from build123d import *

# Parameters (mm, degrees)
F0_R     = 1
F1_DEPTH = 22.5
F2_W     = 4
F2_H     = 5.5
F3_DEPTH = 12.5
F4_W     = 4
F4_H     = 2.8967225653
F4_H_2   = 2.6032774347
F5_DEPTH = 12.5


with BuildPart() as f1:
    # F0 (on Right) → F1 (new body)
    with BuildSketch(Plane.YZ):
        with BuildLine():
            Line((-2.25, 6.0981554588), (-2.4978658434, 0.1032774347))
            ThreePointArc((-2.4978658434, 0.1032774347), (0, -2.5), (2.4978658434, 0.1032774347))
            Line((2.4978658434, 0.1032774347), (2.25, 6.0981554588))
            Line((2.25, 6.0981554588), (-2.25, 6.0981554588))
        make_face()
        Circle(F0_R, mode=Mode.SUBTRACT)
    extrude(amount=F1_DEPTH)

    # F2 (on Front) → F3 (intersect, symmetric)
    with BuildSketch(Plane.XZ):
        Polygon((18.25, 6.0981554588), (4.25, 6.0981554588), (4.25, 4.5981554588), (0.5, 4.5981554588), (0, -2.5), (5.25, -2.5), (5.25, 3), (9.25, 3), (9.25, -2.5), (13.25, -2.5), (13.25, 3), (17.25, 3), (17.25, -2.5), (22.0024140141, -2.5), (22.0008491054, 4.5981554588), (18.25, 4.5981554588), align=None)
        Polygon((5.25, -2.5), (0, -2.5), (5.25, -3.4987433143), align=None)
        Polygon((21.3468169383, -4.6197534539), (22.0024140141, -2.5), (17.25, -2.5), (17.25, -4.6197534539), align=None)
        with Locations((7.25, 0.25)):
            Rectangle(F2_W, F2_H)
        with Locations((15.25, 0.25)):
            Rectangle(F2_W, F2_H)
        Polygon((13.25, -2.5), (9.25, -2.5), (9.25, -3.4987433143), (13.25, -4.6197534539), align=None)
    extrude(amount=F3_DEPTH, both=True, mode=Mode.INTERSECT)

    # F4 (on Front) → F5 (cut, symmetric)
    with BuildSketch(Plane.XZ):
        with Locations((7.25, 1.5516387174)):
            Rectangle(F4_W, F4_H)
        Polygon((9.25, -2.5), (5.25, -2.5), (5.25, -7), (17.25, -7), (17.25, -2.5), (13.25, -2.5), (13.25, -5), (9.25, -5), align=None)
        with Locations((7.25, -1.1983612826)):
            Rectangle(F4_W, F4_H_2)
        with Locations((15.25, 1.5516387174)):
            Rectangle(F4_W, F4_H)
        with Locations((15.25, -1.1983612826)):
            Rectangle(F4_W, F4_H_2)
    extrude(amount=F5_DEPTH, both=True, mode=Mode.SUBTRACT)


solid = f1.part
CAD build for the part. Positions are in the model's coordinates, mm. A direction names the side the tool comes from. Round coordinates to 2 decimals unless told otherwise and drop trailing zeros. Loops run counter-clockwise (first coordinate to the right, second up) from the corner with the lowest first, then second, coordinate; pieces in that order, holes last.
(1) Which spindle directions (+Z, -Z, +X, -X, +Y, -Y) get a long thin tool onto all of the face, cutting with end or side? Do faces 1 (the flat face through (20, 0, 4.598)), 2 (the flat face through (10.94, 2.376, 3.059)), 3 (the flat face through (2, 0, 4.598)), 4 (the flat face through (15, 0, 3)), 5 (the cylindrical face through (11, 0, -1)). Say none if no direction does.
(2) Cut at B-B (z = 2). Give the cut face in (x, y), plus the area to 3 significant figures.
(3) Two-plate mould, pull along X, no slides. Class faces 6 (the flat face through (13.25, -1, 1)), 7 (the flat face through (18.25, 0, 5)), 8 (the cylindrical face through (20, 0, -1)), 9 (the flat face through (17.25, -1, 1)): +X half, -X half, draft (parallel to the pull), parting line (faces both ways), or undercut.
(4) Wall check: line 1 along X through (y, z) = (-0.45, -1); line 2 along Y through (x, z) = (2.5, 0); line 3 along Z through (x, y) = (2.6, 0). Give the ranges that are in metal, low to high.
(5) Drop flat-ended pins along their axis: pin 1 (3 mm diameter, centred on x = 7.5, y = 1, fed in from -Z); pin 2 (2.5 mm diameter, centred on y = 0, z = 0, fed in from -X); pin 3 (1.8 mm diameter, centred on y = 0, z = 0, fed in from -X); pin 4 (0.8 mm diameter, centred on y = -1, z = 5.5, fed in from +X). Give the stop position or say it passes through.
(6) Cut at D-D (y = 1.5). Give the cut face in (x, z), plus the area to 3 significant figures.
(7) Cut at A-A (y = 0.3). Give the cut face in (x, z), plus the area to 3 significant figures.
Findings below:
1. face 1: +Z, +X, +Y, -Y
1. face 2: +Z, +X, -X, +Y
1. face 3: +Z, -X, +Y, -Y
1. face 4: -Z, +Y, -Y
1. face 5: +X, -X
2. outline: (0.32, -2.42) - (5.25, -2.42) - (5.25, 2.42) - (0.32, 2.42) - close; (9.25, -2.42) - (13.25, -2.42) - (13.25, 2.42) - (9.25, 2.42) - close; (17.25, -2.42) - (22, -2.42) - (22, 2.42) - (17.25, 2.42) - close
2. area: 66.2 mm2
3. face 6: undercut
3. face 7: +X half
3. face 8: draft
3. face 9: undercut
4. line 1: x = 0.11 to 5.25, 9.25 to 13.25, 17.25 to 22
4. line 2: y = -2.5 to -1, 1 to 2.5
4. line 3: z = -2.5 to -1, 1 to 4.6
5. pin 1: stops at z = 3
5. pin 2: stops at x = 0.09
5. pin 3: passes through
5. pin 4: stops at x = 18.25
6. outline: (0.04, -2) - (5.25, -2) - (5.25, 3) - (9.25, 3) - (9.25, -2) - (13.25, -2) - (13.25, 3) - (17.25, 3) - (17.25, -2) - (22, -2) - (22, 4.6) - (18.25, 4.6) - (18.25, 6.1) - (4.25, 6.1) - (4.25, 4.6) - (0.5, 4.6) - close
6. area: 124 mm2
7. outline: (0, -2.48) - (5.25, -2.48) - (5.25, -0.95) - (0.11, -0.95) - close; (0.24, 0.95) - (5.25, 0.95) - (5.25, 3) - (9.25, 3) - (9.25, 0.95) - (13.25, 0.95) - (13.25, 3) - (17.25, 3) - (17.25, 0.95) - (22, 0.95) - (22, 4.6) - (18.25, 4.6) - (18.25, 6.1) - (4.25, 6.1) - (4.25, 4.6) - (0.5, 4.6) - close; (9.25, -2.48) - (13.25, -2.48) - (13.25, -0.95) - (9.25, -0.95) - close; (17.25, -2.48) - (22, -2.48) - (22, -0.95) - (17.25, -0.95) - close
7. area: 105 mm2
